from build123d import *

# Parameters (mm, degrees)
SKETCH_1_R             = 5
EXTRUDE_1_DEPTH        = 89
HOLE_WIZARD_M4_2_D     = 3.3
HOLE_WIZARD_M4_2_DEPTH = 11.5
HOLE_WIZARD_M4_2_TIP   = 0.991420021
HOLE_WIZARD_M4_1_D     = 3.3
HOLE_WIZARD_M4_1_DEPTH = 11.5
HOLE_WIZARD_M4_1_TIP   = 0.991420021
CUT_EXTRUDE_START      = 5
SKETCH_7_W             = 26.609090492
SKETCH_7_H             = 30
CUT_EXTRUDE_1_DEPTH    = 2
HOLE_WIZARD_M4_3_D     = 3.3
HOLE_WIZARD_M4_3_DEPTH = 11.5
HOLE_WIZARD_M4_3_TIP   = 0.991420021


with BuildPart() as part:
    # 草图1 → 凸台-拉伸1 (new body)
    with BuildSketch(Plane(origin=(0, 0, 0), x_dir=(1, 0, 0), z_dir=(0, 1, 0))):
        with Locations(Location((0, 0, 0), (0, 0, 270))):
            Circle(SKETCH_1_R)
    extrude(amount=EXTRUDE_1_DEPTH)

    # M4 螺纹孔2
    with Locations(Plane(origin=(0, 89, 0), x_dir=(1, 0, 0), z_dir=(0, 1, 0))):
        with Locations((0, 0)):
            Hole(HOLE_WIZARD_M4_2_D / 2, depth=HOLE_WIZARD_M4_2_DEPTH)
            with Locations((0, 0, -(HOLE_WIZARD_M4_2_DEPTH + HOLE_WIZARD_M4_2_TIP / 2))):  # 118° drill point
                Cone(0, HOLE_WIZARD_M4_2_D / 2, HOLE_WIZARD_M4_2_TIP, mode=Mode.SUBTRACT)

    # M4 螺纹孔1
    with Locations(Plane(origin=(0, 0, 0), x_dir=(-1, 0, 0), z_dir=(0, -1, 0))):
        with Locations((0, 0)):
            Hole(HOLE_WIZARD_M4_1_D / 2, depth=HOLE_WIZARD_M4_1_DEPTH)
            with Locations((0, 0, -(HOLE_WIZARD_M4_1_DEPTH + HOLE_WIZARD_M4_1_TIP / 2))):  # 118° drill point
                Cone(0, HOLE_WIZARD_M4_1_D / 2, HOLE_WIZARD_M4_1_TIP, mode=Mode.SUBTRACT)

    # 草图7 → 切除-拉伸1 (cut)
    with BuildSketch(Plane(origin=(0, 0, 0), x_dir=(0, 0, -1), z_dir=(1, 0, 0)).offset(CUT_EXTRUDE_START)):
        with Locations((0, 40)):
            Rectangle(SKETCH_7_W, SKETCH_7_H)
    extrude(amount=-CUT_EXTRUDE_1_DEPTH, mode=Mode.SUBTRACT)

    # M4 螺纹孔3
    with Locations(Plane(origin=(3, 0, 0), x_dir=(0, 0, -1), z_dir=(1, 0, 0))):
        with Locations((0, 40)):
            Hole(HOLE_WIZARD_M4_3_D / 2, depth=HOLE_WIZARD_M4_3_DEPTH)
            with Locations((0, 0, -(HOLE_WIZARD_M4_3_DEPTH + HOLE_WIZARD_M4_3_TIP / 2))):  # 118° drill point
                Cone(0, HOLE_WIZARD_M4_3_D / 2, HOLE_WIZARD_M4_3_TIP, mode=Mode.SUBTRACT)


solid = part.part
Read the model definition and answer for the solid it produces. Units are mm, in the model's axes. A direction names the side the tool comes from. Coordinates: 2 decimals unless noted, no trailing zeros. Order: outer loops, then holes, each group sorted by start corner. A loop starts at its lowest first (then second) coordinate and runs counter-clockwise, first axis right, second up. Notation, with made-up numbers: (77, 53.25) - (104, 53.25) arc R13 ccw to (104, 60.25) - close; hole circle Ø10 at (63, 72.5). An arc over 180 degrees is marked (long way). Use one line per item in the form item = value.
(1) Section A-A, the plane x = -3 is taken. Give the vertices of the cut face in (y, z), then the cut area to 3 significant figures.
Computed values:
outline = (0, -4) - (89, -4) - (89, 4) - (0, 4) - close; hole circle Ø3.3 at (40, 0)
area = 703 mm²
(2) Straight lines are drawn through the part: L1, parallel to Y at x = -2.5, z = 0; L2, parallel to Z at x = 3, y = 9; L3, parallel to Y at x = -1.5, z = 0.25. For each, find the intervals that lie inside material, in ascending order.
Computed values:
L1 = 0 to 38.35, 41.65 to 89
L2 = -4 to 4
L3 = 11.58 to 38.37, 41.63 to 77.42
(3) Given pin 1 Ø2 at (y, z) = (57.5, -1.5) entering from +X; pin 2 Ø1 at (x, y) = (-1, 29) entering from +Z; pin 3 Ø2 at (x, y) = (2.5, 55.5) entering from +Z, each flat-ended and moving along its own axis, determine where each tip first touches the part or whether it passes through.
Computed values:
pin_1 = 4.97
pin_2 = 4.97
pin_3 = 4.77
(4) Which of the six approach directions +Z, -Z, +X, -X, +Y, -Y give full straight-line access (tool end or side, diameter ignored) to faces 4 (the face through (-1.06, 41.39, 0.89)), 5 (the face through (4, 25, 0)), 6 (the face through (1.216, 83.17, -1.115))?
Computed values:
face_4 = +X, -X
face_5 = +Z, -Z, +X
face_6 = +Y
(5) For a pull along Z with two mould halves and no side action, classify faces 1 (the face through (4, 55, 0)), 2 (the face through (-4.88, 43.88, -1.08)), 3 (the face through (-1.216, 5.831, -1.115)) as pulls with the +Z half, pulls with the -Z half, needs draft (parallel to the pull), parting line crosses it, or undercut.
Computed values:
face_1 = needs draft
face_2 = parting line crosses it
face_3 = undercut
(6) Section D-D, the plane z = 2.5 is taken. Give the vertices of the cut face in (x, y), then the cut area to 3 significant figures.
Computed values:
outline = (-4.33, 0) - (4.33, 0) - (4.33, 25) - (3, 25) - (3, 55) - (4.33, 55) - (4.33, 89) - (-4.33, 89) - close
area = 731 mm²
(7) Section B-B, the plane y = 40 is taken. Give the vertices of the cut face in (x, z).
Computed values:
outline = (-4.72, -1.65) arc R5 ccw to (3, -4) - (3, -1.65) - close; (-4.72, 1.65) - (3, 1.65) - (3, 4) arc R5 ccw to start
(8) Section C-C, the plane y = 9.5 is taken. Give the vertices of the cut face in (x, z), then the cut area to 3 significant figures.
Computed values:
outline = circle Ø10 at (0, 0); hole circle Ø3.3 at (0, 0)
area = 70.0 mm²
